```python
from build123d import *

# Parameters (mm, degrees)
SKETCH3_W           = 300
SKETCH3_H           = 180
BOSS_EXTRUDE2_DEPTH = 3
CUT_EXTRUDE1_DEPTH  = 3
CUT_EXTRUDE2_DEPTH  = 3
CUT_EXTRUDE3_DEPTH  = 10
CUT_EXTRUDE4_DEPTH  = 10
CUT_EXTRUDE5_DEPTH  = 10


with BuildPart() as part:
    # Sketch3 → Boss-Extrude2 (new body)
    with BuildSketch(Plane.XY):
        Rectangle(SKETCH3_W, SKETCH3_H)
    extrude(amount=BOSS_EXTRUDE2_DEPTH)

    # Sketch4 → Cut-Extrude1 (cut)
    with BuildSketch(Plane.XY.offset(3)):
        with BuildLine():
            Line((-140.5, 83), (-140.5, 73))
            ThreePointArc((-140.5, 73), (-142.5, 71), (-144.5, 73))
            Line((-144.5, 73), (-144.5, 83))
            ThreePointArc((-144.5, 83), (-142.5, 85), (-140.5, 83))
        make_face()
        with BuildLine():
            Line((2, 83), (2, 73))
            ThreePointArc((2, 73), (0, 71), (-2, 73))
            Line((-2, 73), (-2, 83))
            ThreePointArc((-2, 83), (0, 85), (2, 83))
        make_face()
        with BuildLine():
            Line((144.5, 83), (144.5, 73))
            ThreePointArc((144.5, 73), (142.5, 71), (140.5, 73))
            Line((140.5, 73), (140.5, 83))
            ThreePointArc((140.5, 83), (142.5, 85), (144.5, 83))
        make_face()
    extrude(amount=-CUT_EXTRUDE1_DEPTH, mode=Mode.SUBTRACT)

    # Sketch5 → Cut-Extrude2 (cut)
    with BuildSketch(Plane.XY.offset(3)):
        with BuildLine():
            Line((-143, 2), (-133, 2))
            ThreePointArc((-133, 2), (-131, 0), (-133, -2))
            Line((-133, -2), (-143, -2))
            ThreePointArc((-143, -2), (-145, 0), (-143, 2))
        make_face()
        with BuildLine():
            Line((133, 2), (143, 2))
            ThreePointArc((143, 2), (145, 0), (143, -2))
            Line((143, -2), (133, -2))
            ThreePointArc((133, -2), (131, 0), (133, 2))
        make_face()
    extrude(amount=-CUT_EXTRUDE2_DEPTH, mode=Mode.SUBTRACT)

    # Sketch6 → Cut-Extrude3 (cut)
    with BuildSketch(Plane.XY.offset(3)):
        with BuildLine():
            Line((143, -84.5), (133, -84.5))
            ThreePointArc((133, -84.5), (131, -82.5), (133, -80.5))
            Line((133, -80.5), (143, -80.5))
            ThreePointArc((143, -80.5), (145, -82.5), (143, -84.5))
        make_face()
    extrude(amount=-CUT_EXTRUDE3_DEPTH, mode=Mode.SUBTRACT)

    # Sketch7 → Cut-Extrude4 (cut)
    with BuildSketch(Plane.XY.offset(3)):
        with BuildLine():
            Line((-143, -80.5), (-133, -80.5))
            ThreePointArc((-133, -80.5), (-131, -82.5), (-133, -84.5))
            Line((-133, -84.5), (-143, -84.5))
            ThreePointArc((-143, -84.5), (-145, -82.5), (-143, -80.5))
        make_face()
    extrude(amount=-CUT_EXTRUDE4_DEPTH, mode=Mode.SUBTRACT)

    # Sketch8 → Cut-Extrude5 (cut)
    with BuildSketch(Plane.XY.offset(3)):
        with BuildLine():
            Line((-120, -46), (120, -46))
            ThreePointArc((120, -46), (122, -48), (120, -50))
            Line((120, -50), (-120, -50))
            ThreePointArc((-120, -50), (-122, -48), (-120, -46))
        make_face()
    extrude(amount=-CUT_EXTRUDE5_DEPTH, mode=Mode.SUBTRACT)


solid = part.part
```
The model under review builds one solid part; all positions refer to its coordinate system, in mm. Round coordinates to 2 decimals unless told otherwise and drop trailing zeros. Order: outer loops, then holes, each group sorted by start corner. A loop starts at its lowest first (then second) coordinate and runs counter-clockwise, first axis right, second up.
(1) Wall thickness on L1, parallel to Y at x = 22, z = 2.1; L2, parallel to X at y = -46.5, z = 2.35: over which ranges is each line inside the solid? List them lowest first.
Working result:
L1: y = -90 to -50, -46 to 90
L2: x = -150 to -121.32, 121.32 to 150
(2) Take a section at A-A, the plane x = -37. State the section outline as (y, z) points.
Working result:
outline: (-90, 0) - (-50, 0) - (-50, 3) - (-90, 3) - close; (-46, 0) - (90, 0) - (90, 3) - (-46, 3) - close
(3) Take a section at B-B, the plane z = 1.6. Count the separate pieces of the cut face and the enclosed holes in it, plus the area to 3 significant figures.
Working result:
separate pieces: 1
enclosed holes: 8
area: 52,700 mm2
